from build123d import *

# Parameters (mm, degrees)
F0_R     = 24.2
F1_DEPTH = 30
F2_R     = 5
F3_DEPTH = 25
F4_R     = 5


with BuildPart() as f1:
    # F0 (on Front) → F1 (new body)
    with BuildSketch(Plane.XZ):
        with BuildLine():
            Line((24, 60), (24, 16.278821))
            ThreePointArc((24, 16.278821), (-27.721833, -8.514693), (29, 0))
            Line((29, 0), (29, 60))
            Line((29, 60), (24, 60))
        make_face()
        Circle(F0_R, mode=Mode.SUBTRACT)
    extrude(amount=F1_DEPTH)

    # F2 (on face) → F3 (cut)
    with BuildSketch(Plane.YZ.offset(29)):
        with Locations((-15, 48)):
            Circle(F2_R)
    extrude(amount=-F3_DEPTH, mode=Mode.SUBTRACT)

    # F4
    f4_edges = [f1.edges().sort_by_distance(p)[0] for p in [
        (24, -15, 16.278821),
        (26.5, -30, 60),
        (26.5, 0, 60),
    ]]
    fillet(f4_edges, radius=F4_R)


solid = f1.part
Here's how the part is built. I have some questions about the finished solid (model axes, mm). Coordinates: 2 decimals unless noted, no trailing zeros. Order: outer loops, then holes, each group sorted by start corner. A loop starts at its lowest first (then second) coordinate and runs counter-clockwise, first axis right, second up.
Item 1: If we mould it in two halves opening along X, with no side actions, what happens to faces 1 (the face through (26, -2, 59)), 2 (the face through (29, -15, 30)), 3 (the face through (21.415, -15.21, 23.818)), 4 (the face through (22.355, -14.79, -9.269))? For each: +X half, -X half, draft (parallel to the pull), parting line (faces both ways), or undercut.
Result sheet:
face 1: draft
face 2: +X half
face 3: undercut
face 4: undercut
Item 2: If we section it at D-D on y = -3.5: List the corners of the cut face in (x, z) for me, plus the area to 3 significant figures.
Result sheet:
outline: (16.21, 24.05) arc R29 ccw (long way) to (29, 0) - (29, 59.77) - (24, 59.77) - (24, 28.2) arc R5 cw to start; hole circle Ø48.4 at (0, 0)
area: 1,070 mm2
Item 3: If we section it at B-B on z = -4: List the corners of the cut face in (x, y) for me.
Result sheet:
outline: (-28.72, -30) - (-23.87, -30) - (-23.87, 0) - (-28.72, 0) - close; (23.87, -30) - (28.72, -30) - (28.72, 0) - (23.87, 0) - close
Item 4: For P1, Ø3, axis at x = -2.5, y = -15.5, coming from the +Z side; P2, Ø16, axis at y = -15, z = 48, coming from the -X side; P3, Ø2, axis at y = -24, z = 7, coming from the -X side, each with a flat end and sliding along its axis, tell me the tip position at first contact or that it passes through.
Result sheet:
P1: stops at z = 28.98
P2: stops at x = 24
P3: stops at x = -28.37
Item 5: I need wall thicknesses on line 1 (Z direction, x = 0, y = -18.75); line 2 (X direction, y = -9.5, z = 30); line 3 (Z direction, x = 9, y = -2). Which ranges of each line are inside material? Lowest first, please.
Result sheet:
line 1: z = -29 to -24.2, 24.2 to 29
line 2: x = 24 to 29
line 3: z = -27.57 to -22.46, 22.46 to 27.57
Item 6: If we section it at A-A on y = -12.75: List the corners of the cut face in (x, z) for me, plus the area to 3 significant figures.
Result sheet:
outline: (16.21, 24.05) arc R29 ccw (long way) to (29, 0) - (29, 43.53) - (24, 43.53) - (24, 28.2) arc R5 cw to start; (24, 52.47) - (29, 52.47) - (29, 60) - (24, 60) - close; hole circle Ø48.4 at (0, 0)
area: 1,030 mm2
Item 7: If we section it at C-C on x = 0: List the corners of the cut face in (y, z) for me.
Result sheet:
outline: (-30, -29) - (0, -29) - (0, -24.2) - (-30, -24.2) - close; (-30, 24.2) - (0, 24.2) - (0, 29) - (-30, 29) - close
